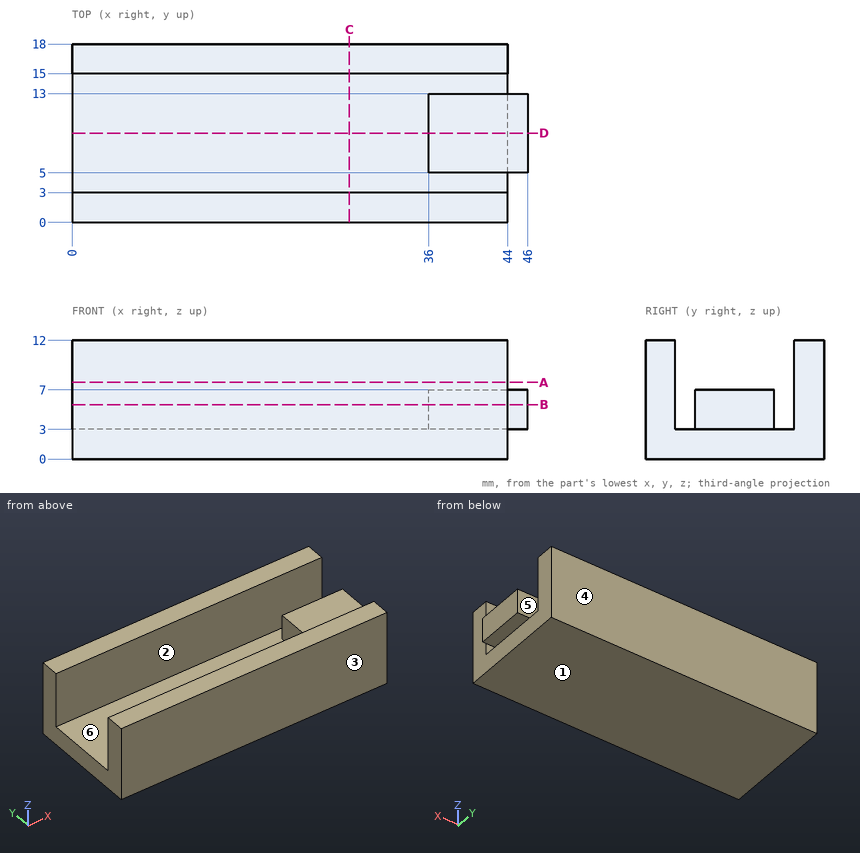
Verification items for this drawing (mm, ordinates from the low corner). A direction names the side the tool comes from. Coordinates: 2 decimals unless noted, no trailing zeros. Order: outer loops, then holes, each group sorted by start corner. A loop starts at its lowest first (then second) coordinate and runs counter-clockwise, first axis right, second up. Notation, with made-up numbers: M 7,45.5 L 13,45.5 A22 cw 13,77.5 Z; hole C 54,79 d4. An arc over 180 degrees is marked long. One line per item, written item: value. Start each with the question number.
Item 1: Sectioned sample at C-C on x = 28. Record the cut outline in (y, z).
Item 2: Sectioned sample at A-A on z = 7.75. Record the cut outline in (x, y).
Item 3: Sectioned sample at B-B on z = 5.5. Record the cut outline in (x, y), then the cut area to 3 significant figures.
Item 4: Sectioned sample at D-D on y = 9. Record the cut outline in (x, z).
Item 5: Thickness scan on probe 1 along Y at (x, z) = (41, 6.5); probe 2 along Y at (x, z) = (21, 7.75); probe 3 along X at (y, z) = (16.75, 9.5). Record the ranges inside material, lowest first.
Item 6: Access from +Z, -Z, +X, -X, +Y, -Y to the whole of each face (thin tool, end or side, straight path). Record for the marked faces 1 and 2.
Item 7: Mould release check, pull along Y, two halves, no side actions. Record for the marked faces 3, 4, 5 and 6: pulls with the +Y half, pulls with the -Y half, needs draft (parallel to the pull), parting line crosses it, or undercut.
Item 8: Depth check by flat-ended pin: P1, Ø3, axis at y = 12.5, z = 5, coming from the -X side; P2, Ø7, axis at x = 26.5, z = 9.5, coming from the -Y side; P3, Ø6.5, axis at x = 41.5, y = 7.5, coming from the +Z side; P4, Ø3, axis at x = 10.5, y = 5.5, coming from the +Z side. Enter the tip coordinate at first touch or a pass-through.
Calculated:
1. outline: M 0,0 L 18,0 L 18,12 L 15,12 L 15,3 L 3,3 L 3,12 L 0,12 Z
2. outline: M 0,0 L 44,0 L 44,3 L 0,3 Z; M 0,15 L 44,15 L 44,18 L 0,18 Z
3. outline: M 0,0 L 44,0 L 44,3 L 0,3 Z; M 0,15 L 44,15 L 44,18 L 0,18 Z; M 36,5 L 46,5 L 46,13 L 36,13 Z
3. area: 344 mm^2
4. outline: M 0,0 L 44,0 L 44,3 L 46,3 L 46,7 L 36,7 L 36,3 L 0,3 Z
5. probe 1: 0 to 3, 5 to 13, 15 to 18
5. probe 2: 0 to 3, 15 to 18
5. probe 3: 0 to 44
6. face 1: -Z, +X, -X, +Y, -Y
6. face 2: +Z, +X, -X
7. face 3: pulls with the -Y half
7. face 4: pulls with the +Y half
7. face 5: undercut
7. face 6: undercut
8. P1: x = 36
8. P2: y = 0
8. P3: z = 7
8. P4: z = 3
